Source: CAD feature listing. Evaluate the final solid. Frame: model axes, mm. A direction names the side the tool comes from. Coordinates: 2 decimals unless noted, no trailing zeros. Write each loop counter-clockwise with the first axis right and the second up, starting at its lowest first coordinate (ties: lowest second). Pieces come first, ordered by that corner, then holes. Notation, with made-up numbers: M -3,8 L 22,8 A33 ccw 22,38 Z; hole C 87,-36.5 d6. An arc over 180 degrees is marked long. Answer as CSV lines item,"result". Start each with the question number.
1. Mould query, pull axis X, two halves, no side actions, for faces 1 (the face through (-6.3, 1.5, -53.8)), 2 (the face through (-200, -3, -40)), 3 (the face through (-33.87, -10.23, -53.55)). Classes: pulls with the +X half, pulls with the -X half, needs draft (parallel to the pull), parting line crosses it, or undercut.
2. Line query: probe 1 along Z at (x, y) = (-30, -8.75); probe 2 along X at (y, z) = (-0.5, -30); probe 3 along X at (y, z) = (-11, -53). Output: solid intervals per line, ascending. Write a range as [from, to].
3. Reachability of faces 4 (the face through (-152.5, -3, -65)), 5 (the face through (-27, -10, -30)), 6 (the face through (-83, -3, -20)) from +Z, -Z, +X, -X, +Y, -Y: full face, straight path, thin tool, end or side. Return the list, or none.
4. Section B-B on x = -17.5. Return the cut outline in (y, z).
5. Section C-C on x = -144.5. Return the cut outline in (y, z).
6. Section A-A on y = -2. Count the separate pieces of the cut face and the enclosed holes in it, plus the area to 3 significant figures.
7. Contact query for flat-ended pins moving along their axis: pin 1 Ø1.7 at (y, z) = (-11, -29.5) entering from +X; pin 2 Ø6 at (y, z) = (-9.5, -29.5) entering from +X; pin 3 Ø4 at (x, z) = (-162.5, -72.5) entering from -Y. Output: stop coordinate, or through.
Autodesk Inventor part; units mm, degrees
ref_plane "Work Plane1" through (0, -2.75, 0) normal (0, -1, 0) x (1, 0, 0)
ref_plane "Work Plane2" through (-152.5, -8.5, -20) normal (0, 0, -1) x (-1, 0, 0)
ref_plane "Work Plane3" through (-152.5, -8.5, -40) normal (0, 0, -1) x (-1, 0, 0)
sketch "Sketch1" plane through (0, 0, 0) normal (0, 1, 0) x (-1, 0, 0)
  line L0 (0, 0) -> (200, 0)
  line L1 (200, 0) -> (200, -80)
  line L2 (200, -80) -> (0, -80)
  line L3 (0, -80) -> (0, 0)
  line L4 (10, -30) -> (30, -30)
  line L5 (30, -30) -> (30, -50)
  line L6 (30, -50) -> (10, -50)
  line L7 (10, -50) -> (10, -30)
  circle A0 centre (10, -30) radius 1.5
  circle A1 centre (30, -50) radius 1.5
  circle A2 centre (30, -30) radius 1.5
  circle A3 centre (10, -50) radius 1.5
  line L8 (192.5, -7.5) -> (162.5, -7.5)
  line L9 (162.5, -7.5) -> (162.5, -72.5)
  line L10 (162.5, -72.5) -> (192.5, -72.5)
  line L11 (192.5, -72.5) -> (192.5, -7.5)
  circle A4 centre (192.5, -7.5) radius 1.5
  circle A5 centre (192.5, -72.5) radius 1.5
  circle A6 centre (162.5, -72.5) radius 1.5
  circle A7 centre (162.5, -7.5) radius 1.5
  line L12 (200, 0) -> (152.5, 0)
  line L13 (152.5, 0) -> (152.5, -80)
  line L14 (152.5, -80) -> (200, -80)
  line L15 (200, -80) -> (200, 0)
  line L16 (152.5, -20) -> (0, -20)
  line L17 (0, -20) -> (0, -60)
  line L18 (0, -60) -> (152.5, -60)
  line L19 (152.5, -60) -> (152.5, -20)
  line L20 (40, -20) -> (40, -60)
  point P0 (191, -7.5)
  point P1 (192.5, -9)
  point P2 (192.5, -71)
  point P3 (191, -72.5)
  point P4 (164, -72.5)
  point P5 (162.5, -71)
  point P6 (164, -7.5)
  point P7 (162.5, -9)
  point P8 (152.5, 0)
  point P9 (0, -20)
  dimension "d0" = 200
  dimension "d1" = 80
  dimension "d2" = 20
  dimension "d3" = 20
  dimension "d4" = 30
  dimension "d5" = 10
  dimension "d6" = 3
  dimension "d7" = 3
  dimension "d8" = 3
  dimension "d9" = 3
  dimension "d10" = 65
  dimension "d11" = 30
  dimension "d12" = 7.5
  dimension "d13" = 7.5
  dimension "d14" = 3
  dimension "d15" = 3
  dimension "d16" = 3
  dimension "d17" = 3
  dimension "d18" = 20
  dimension "d19" = 20
  dimension "d20" = 10
  dimension "d23" = 40
extrude "Extrusion1" add sketch "Sketch1" along normal blind 3 contours L0 L1 L2 L13 | L16 L20 L18 L3 | L13 L18 L20 L16 | L4 A2 L5 A1 L6 A3 L7 A0 | L8 A4 L11 A5 L10 A6 L9 A7
extrude "Extrusion2" add sketch "Sketch1" against normal blind 5.5 contours L0 L1 L2 L13 | L13 L18 L20 L16 | L8 A4 L11 A5 L10 A6 L9 A7
ref_plane "Work Plane1" through (0, -2.75, 0) normal (0, -1, 0) x (1, 0, 0)
mirror "Mirror1" about plane through (0, -2.75, 0) normal (0, -1, 0) of "Extrusion1"
chamfer "Chamfer1" distance 12.5 angle 45 4 edges at (0, 1.5, -20) (0, -7, -20) (0, -7, -60) (0, 1.5, -60)
ref_plane "Work Plane2" through (-152.5, -8.5, -20) normal (0, 0, -1) x (-1, 0, 0)
fillet "Fillet2" radius 10 4 edges at (-200, -2.75, -80) (-152.5, -2.75, -80) (-152.5, -2.75, 0) (-200, -2.75, 0)
sketch "Sketch5" plane through (-152.5, -8.5, -60) normal (0, -1, 0) x (1, 0, 0)
  circle A0 centre (122.5, 30) radius 1.5
  line L0 (122.5, 33.4641) -> (125.5, 31.7321)
  line L1 (125.5, 31.7321) -> (125.5, 28.2679)
  line L2 (125.5, 28.2679) -> (122.5, 26.5359)
  line L3 (122.5, 26.5359) -> (119.5, 28.2679)
  line L4 (119.5, 28.2679) -> (119.5, 31.7321)
  line L5 (119.5, 31.7321) -> (122.5, 33.4641)
  circle A1 centre (142.5, 30) radius 1.5
  line L6 (142.5, 33.4641) -> (145.5, 31.7321)
  line L7 (145.5, 31.7321) -> (145.5, 28.2679)
  line L8 (145.5, 28.2679) -> (142.5, 26.5359)
  line L9 (142.5, 26.5359) -> (139.5, 28.2679)
  line L10 (139.5, 28.2679) -> (139.5, 31.7321)
  line L11 (139.5, 31.7321) -> (142.5, 33.4641)
  circle A2 centre (142.5, 10) radius 1.5
  line L12 (142.5, 13.4641) -> (145.5, 11.7321)
  line L13 (145.5, 11.7321) -> (145.5, 8.2679)
  line L14 (145.5, 8.2679) -> (142.5, 6.5359)
  line L15 (142.5, 6.5359) -> (139.5, 8.2679)
  line L16 (139.5, 8.2679) -> (139.5, 11.7321)
  line L17 (139.5, 11.7321) -> (142.5, 13.4641)
  circle A3 centre (122.5, 10) radius 1.5
  line L18 (122.5, 13.4641) -> (125.5, 11.7321)
  line L19 (125.5, 11.7321) -> (125.5, 8.2679)
  line L20 (125.5, 8.2679) -> (122.5, 6.5359)
  line L21 (122.5, 6.5359) -> (119.5, 8.2679)
  line L22 (119.5, 8.2679) -> (119.5, 11.7321)
  line L23 (119.5, 11.7321) -> (122.5, 13.4641)
  circle A4 centre (122.5, 30) radius 5.25
  circle A5 centre (142.5, 30) radius 5.25
  circle A6 centre (142.5, 10) radius 5.25
  circle A7 centre (122.5, 10) radius 5.25
  point P0 (152.5, 60)
  dimension "d44" = 6
  dimension "d45" = 6
  dimension "d46" = 6
  dimension "d47" = 6
  dimension "d48" = 10.5
  dimension "d49" = 10.5
  dimension "d50" = 10.5
  dimension "d51" = 10.5
extrude "Extrusion5" add sketch "Sketch5" along normal blind 3.5 contours A4 | A5 | A6 | A7
sketch "Sketch6" plane through (-152.5, -8.5, -60) normal (0, -1, 0) x (1, 0, 0)
  circle A0 centre (35, 10) radius 1.5
  line L0 (140, 0) -> (0, 0)
  line L1 (0, 0) -> (0, -10)
  circle A1 centre (55, 10) radius 1.5
  circle A2 centre (75, 10) radius 1.5
  circle A3 centre (95, 10) radius 1.5
  point P0 (152.5, 60)
  dimension "d54" = 3
  dimension "d55" = 10
  dimension "d56" = 35
  dimension "d59" = 20
extrude "Extrusion6" cut sketch "Sketch6" against normal blind 33.25
ref_plane "Work Plane3" through (-152.5, -8.5, -40) normal (0, 0, -1) x (-1, 0, 0)
mirror "Mirror2" about plane through (-152.5, -8.5, -40) normal (0, 0, -1) of "Extrusion6"
properties part number "RobotBaseMotorExt"
Values:
1,face 1,"pulls with the +X half"
1,face 2,"pulls with the -X half"
1,face 3,"undercut"
2,probe 1,"[-55.25, -53.46], [-46.54, -44.75], [-35.25, -33.46], [-26.54, -24.75]"
2,probe 2,"[-200, -119], [-116, -99], [-96, -79], [-76, -59], [-56, -40]"
2,probe 3,"[-34.31, -30.8], [-29.2, -25.69], [-14.31, -10.8], [-9.2, -5.69]"
3,face 4,"-Z, +X, +Y, -Y"
3,face 5,"-Y"
3,face 6,"+Z, +X, +Y, -Y"
4,outline,"M -8.5,-60 L -5.5,-60 L -5.5,-20 L -8.5,-20 Z; M 0,-60 L 3,-60 L 3,-20 L 0,-20 Z"
5,outline,"M -8.5,-60 L 3,-60 L 3,-20 L -8.5,-20 Z"
6,separate pieces,"1"
6,enclosed holes,"12"
6,area,"8,130 mm²"
7,pin 1,"x = -4.75"
7,pin 2,"x = -0.17"
7,pin 3,"y = -8.5"
